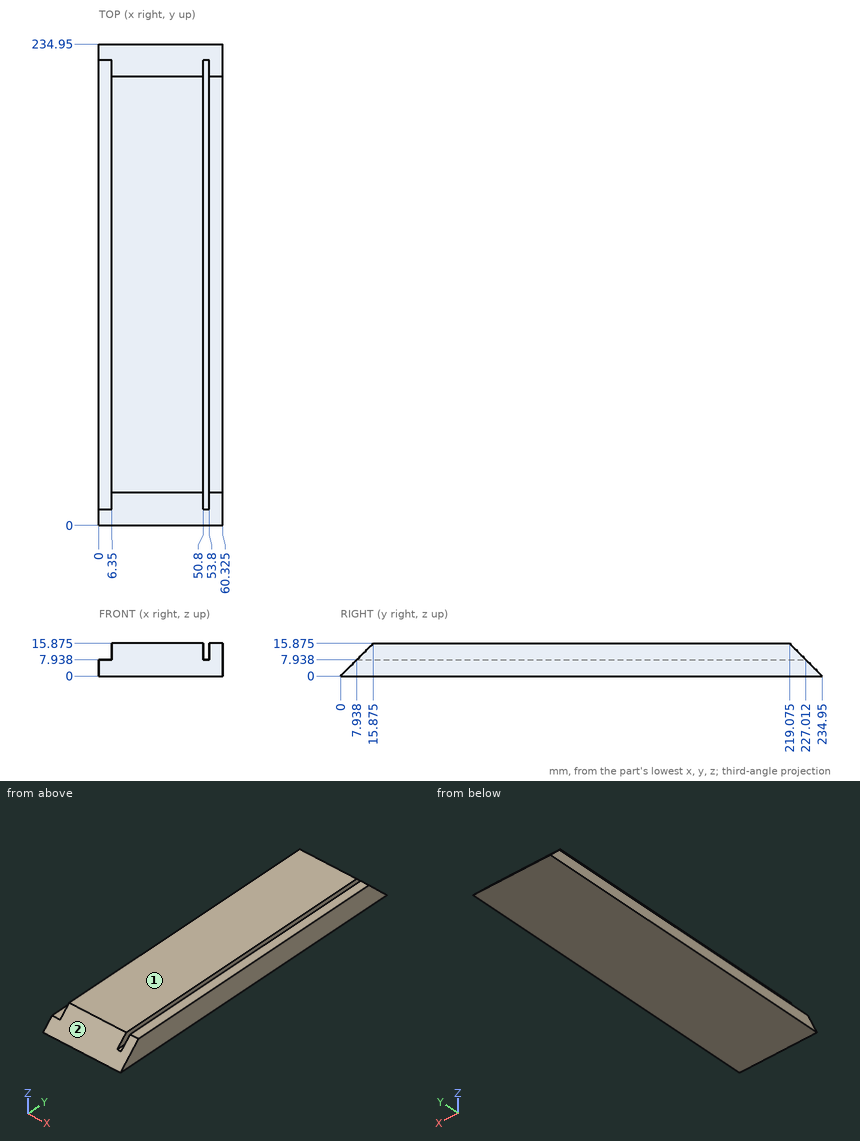
Could you check a few things on this drawing? It's one solid part, dimensions in mm from its lowest x, y, z. Coordinates: 2 decimals unless noted, no trailing zeros.
1. Thinking about a two-plate mould opening in Y: for the marked faces 1 and 2, which applies, +Y half, -Y half, draft (parallel to the pull), parting line (faces both ways), or undercut?
2. I need wall thicknesses on line 1 (Z direction, x = 53, y = 9); line 2 (Y direction, x = 38, z = 10.25); line 3 (Y direction, x = 24.5, z = 12). Which ranges of each line are inside material? Lowest first, please.
3. I'm going to push flat-ended pins straight in: pin 1 (4 mm diameter, centred on y = 103, z = 10, fed in from -X); pin 2 (3 mm diameter, centred on x = 48, z = 2.5, fed in from +Y); pin 3 (1.5 mm diameter, centred on x = 52.5, y = 165.5, fed in from +Z). Where does each tip first touch, or does it pass through?
Entries:
1. face 1: draft
1. face 2: -Y half
2. line 1: z = 0 to 7.94
2. line 2: y = 10.25 to 224.7
2. line 3: y = 12 to 222.95
3. pin 1: stops at x = 6.35
3. pin 2: stops at y = 233.95
3. pin 3: stops at z = 7.94
